Verification items for the finished model (mm, model axes). A direction names the side the tool comes from. Coordinates: 2 decimals unless noted, no trailing zeros. Write each loop counter-clockwise with the first axis right and the second up, starting at its lowest first coordinate (ties: lowest second). Pieces come first, ordered by that corner, then holes. Notation, with made-up numbers: (-26.5, 51) - (3.5, 51) arc R25 cw to (3.5, 64) - close; hole circle Ø1 at (79, 48.25). An arc over 180 degrees is marked (long way). Answer as CSV lines item,"result". Start each with the question number.
```python
from build123d import *

# Parameters (mm, degrees)
SKETCH1_W           = 50
SKETCH1_H           = 50
SKETCH1_W_2         = 40
SKETCH1_H_2         = 40
BOSS_EXTRUDE1_DEPTH = 25
SKETCH2_R           = 3.5
CUT_EXTRUDE1_DEPTH  = 55
SKETCH3_R           = 3.5
CUT_EXTRUDE2_DEPTH  = 55
CUT_EXTRUDE3_DEPTH  = 62.23724357


with BuildPart() as part:
    # Sketch1 → Boss-Extrude1 (new body)
    with BuildSketch(Plane(origin=(0, 0, 0), x_dir=(1, 0, 0), z_dir=(0, 1, 0))):
        Rectangle(SKETCH1_W, SKETCH1_H)
        Rectangle(SKETCH1_W_2, SKETCH1_H_2, mode=Mode.SUBTRACT)
    extrude(amount=BOSS_EXTRUDE1_DEPTH)

    # Sketch2 → Cut-Extrude1 (cut)
    with BuildSketch(Plane(origin=(25, 0, 0), x_dir=(0, 0, -1), z_dir=(1, 0, 0))):
        with Locations((0, 12.5)):
            Circle(SKETCH2_R)
    extrude(amount=-CUT_EXTRUDE1_DEPTH, mode=Mode.SUBTRACT)

    # Sketch3 → Cut-Extrude2 (cut)
    with BuildSketch(Plane.XY.offset(25)):
        with Locations((0, 12.5)):
            Circle(SKETCH3_R)
    extrude(amount=-CUT_EXTRUDE2_DEPTH, mode=Mode.SUBTRACT)

    # Sketch4 → Cut-Extrude3 (cut, through all)
    with BuildSketch(Plane.XY.offset(25)):
        with BuildLine():
            Line((7.5, 25), (25, 25))
            Line((25, 25), (25, 0))
            Line((25, 0), (7.5, 0))
            ThreePointArc((7.5, 0), (20, 12.5), (7.5, 25))
        make_face()
    extrude(amount=-CUT_EXTRUDE3_DEPTH, mode=Mode.SUBTRACT)


solid = part.part
```
1. Cross-section at C-C (y = 12.5). Record the cut outline in (x, z).
2. Depth check by flat-ended pin: P1, Ø7.5, axis at y = 6.5, z = 8.5, coming from the +X side. Enter the tip coordinate at first touch or a pass-through.
3. Cross-section at D-D (x = 0). Record the cut outline in (y, z), and give its area (3 significant figures).
4. Cross-section at A-A (x = -17.5). Record the cut outline in (y, z), and give its area (3 significant figures).
5. Draft check along Y on faces 1 (the face through (-3, 10, 25)), 2 (the face through (19.997, 12.225, 22.535)), 3 (the face through (-0.759, 9.083, -22.465)), 4 (the face through (-22.465, 9.083, 0.759)). Enter one of: pulls with the +Y half, pulls with the -Y half, needs draft (parallel to the pull), parting line crosses it, or undercut.
6. Access from +Z, -Z, +X, -X, +Y, -Y to the whole of each face (thin tool, end or side, straight path). Record for faces 5 (the face through (-20, 12, 5)), 6 (the face through (19.997, 12.225, -22.465)).
7. Cross-section at B-B (z = 0). Record the cut outline in (x, y), and give its area (3 significant figures).
8. Scan lines: line 1 along Z through (x, y) = (-15, 21.25); line 2 along Y through (x, z) = (0, 23); line 3 along X through (y, z) = (21.5, -14). Record each from-to range of solid material in increasing order. Write a range as from..to.
Completed:
1,outline,"(-25, -25) - (-3.5, -25) - (-3.5, -20) - (-20, -20) - (-20, -3.5) - (-25, -3.5) - close; (-25, 3.5) - (-20, 3.5) - (-20, 20) - (-3.5, 20) - (-3.5, 25) - (-25, 25) - close; (3.5, -25) - (20, -25) - (20, -20) - (3.5, -20) - close; (3.5, 20) - (20, 20) - (20, 25) - (3.5, 25) - close"
2,P1,"stops at x = -20"
3,outline,"(0, -25) - (9, -25) - (9, -20) - (0, -20) - close; (0, 20) - (9, 20) - (9, 25) - (0, 25) - close; (16, -25) - (25, -25) - (25, -20) - (16, -20) - close; (16, 20) - (25, 20) - (25, 25) - (16, 25) - close"
3,area,"180 mm2"
4,outline,"(0, -25) - (25, -25) - (25, -20) - (0, -20) - close; (0, 20) - (25, 20) - (25, 25) - (0, 25) - close"
4,area,"250 mm2"
5,face 1,"needs draft"
5,face 2,"parting line crosses it"
5,face 3,"undercut"
5,face 4,"undercut"
6,face 5,"+X, +Y, -Y"
6,face 6,"+Z, -Z, +X"
7,outline,"(-25, 0) - (-20, 0) - (-20, 9) - (-25, 9) - close; (-25, 16) - (-20, 16) - (-20, 25) - (-25, 25) - close"
7,area,"90.0 mm2"
8,line 1,"z = -25..-20, 20..25"
8,line 2,"y = 0..9, 16..25"
8,line 3,"x = -25..-20"
